Source: CAD feature listing. Evaluate the final solid. Frame: model axes, mm. A direction names the side the tool comes from. Give positions to 0.01 mm unless a question says otherwise; leave off trailing zeros. Order: outer loops, then holes, each group sorted by start corner. A loop starts at its lowest first (then second) coordinate and runs counter-clockwise, first axis right, second up. Notation, with made-up numbers: (45.25, 51) -> (103.25, 51) arc R27 ccw to (103.25, 90) -> close; hole circle Ø8 at (69, -10.75). An arc over 180 degrees is marked (long way). Answer in a Markdown table with one row per item.
```python
from build123d import *

# Parameters (mm, degrees)
PAD_DEPTH    = 2
SKETCH_W     = 5.04
SKETCH_H     = 6
POCKET_DEPTH = 2.5


with BuildPart() as part:
    # CopySketch004 → Pad (new body, symmetric)
    with BuildSketch(Plane.XY):
        with BuildLine():
            Line((-36.508492, 11.060009), (-1.723702, 11.060009))
            ThreePointArc((-1.723702, 11.060009), (7.733856, 14.212769), (13.407871, 22.409771))
            Line((13.407871, 22.409771), (24.319128, 59.832547))
            Line((24.319128, 59.832547), (51.226102, 59.832547))
            Line((51.226102, 59.832547), (51.226102, -16.067453))
            Line((24.319128, -16.067453), (51.226102, -16.067453))
            Line((23.401691, -4.060687), (24.319128, -16.067453))
            ThreePointArc((23.401691, -4.060687), (22.843077, -1.909417), (21.705474, 0))
            Line((16, 0), (21.705474, 0))
            Line((16, -10), (16, 0))
            Line((-16, -10), (16, -10))
            Line((-16, -10), (-36.508492, -0.144815))
            Line((-36.508492, 2.549264), (-36.508492, -0.144815))
            Line((-26.508492, 2.549264), (-36.508492, 2.549264))
            Line((-26.508492, 6.549264), (-26.508492, 2.549264))
            Line((-36.508492, 6.549264), (-26.508492, 6.549264))
            Line((-36.508492, 11.060009), (-36.508492, 6.549264))
        make_face()
    extrude(amount=PAD_DEPTH, both=True)

    # Sketch (on Face19 of Pad) → Pocket (cut)
    with BuildSketch(Plane.XY.offset(2)):
        with Locations((0, -7)):
            Rectangle(SKETCH_W, SKETCH_H)
    extrude(amount=-POCKET_DEPTH, mode=Mode.SUBTRACT)


solid = part.part
```
(1) Pull-direction query (Y, two-part tool) for faces 5 (the flat face through (19, 0, 0)), 6 (the flat face through (-26.508, 5, 0)), 7 (the flat face through (2.52, -7, 1)); classes: +Y half, -Y half, draft (parallel to the pull), parting line (faces both ways), or undercut.
A:
| item | result |
|---|---|
| face 5 | -Y half |
| face 6 | undercut |
| face 7 | draft |
(2) Access query for faces 1 (the flat face through (23.854, -9.98, 0.028)), 2 (the flat face through (-2.52, -7, 1)), 3 (the flat face through (0, -10, -1)), 4 (the flat face through (-32, 6.549, 0)). Directions: +Z, -Z, +X, -X, +Y, -Y. A direction counts if a zero-diameter tool reaches every point of the face in a straight line with its end or side. Return the directions, or none.
A:
| item | result |
|---|---|
| face 1 | +Z, -Z, -Y |
| face 2 | +Z, -Y |
| face 3 | +Z, -Z, -X, -Y |
| face 4 | +Z, -Z, -X |
(3) First-contact query: pin 1 Ø1.2 at (x, z) = (-19.5, 0.5) entering from +Y; pin 2 Ø0.8 at (x, z) = (-1, 1) entering from -Y; pin 3 Ø1.2 at (x, z) = (18, 1) entering from -Y. Flat tips, straight axial feed; report the tip coordinate or a pass-through.
A:
| item | result |
|---|---|
| pin 1 | stops at y = 11.06 |
| pin 2 | stops at y = -4 |
| pin 3 | stops at y = 0 |
(4) Section query C-C (y = 38.5). Return the cut outline in (x, z), plus the area to 3 significant figures.
A:
| item | result |
|---|---|
| outline | (18.1, -2) -> (51.23, -2) -> (51.23, 2) -> (18.1, 2) -> close |
| area | 133 mm^2 |
(5) Section query A-A (z = 0.5). Return the cut outline in (x, y), plus the area to 3 significant figures.
A:
| item | result |
|---|---|
| outline | (-36.51, -0.14) -> (-16, -10) -> (-2.52, -10) -> (-2.52, -4) -> (2.52, -4) -> (2.52, -10) -> (16, -10) -> (16, 0) -> (21.71, 0) arc R7.87 cw to (23.4, -4.06) -> (24.32, -16.07) -> (51.23, -16.07) -> (51.23, 59.83) -> (24.32, 59.83) -> (13.41, 22.41) arc R15.76 cw to (-1.72, 11.06) -> (-36.51, 11.06) -> (-36.51, 6.55) -> (-26.51, 6.55) -> (-26.51, 2.55) -> (-36.51, 2.55) -> close |
| area | 3,450 mm^2 |
(6) Section query B-B (x = -8). Return the cut outline in (y, z).
A:
| item | result |
|---|---|
| outline | (-10, -2) -> (11.06, -2) -> (11.06, 2) -> (-10, 2) -> close |
(7) Ray query, probe 1 along X at (y, z) = (-7.5, 1.8); probe 2 along X at (y, z) = (-3.5, 0.9); probe 3 along X at (y, z) = (-1, -1.1). Return the intervals inside material, ascending.
A:
| item | result |
|---|---|
| probe 1 | x = -21.2 to -2.52, 2.52 to 16, 23.66 to 51.23 |
| probe 2 | x = -29.53 to 16, 23.32 to 51.23 |
| probe 3 | x = -34.73 to 16, 22.39 to 51.23 |
